from build123d import *

# Parameters (mm, degrees)
SKETCH1_W           = 48.5
SKETCH1_H           = 28
SKETCH1_W_2         = 40.5
SKETCH1_H_2         = 20
BOSS_EXTRUDE1_DEPTH = 40
SKETCH2_W           = 48.5
SKETCH2_H           = 28
BOSS_EXTRUDE2_DEPTH = 7
SKETCH3_W           = 15
SKETCH3_H           = 15
CUT_EXTRUDE1_DEPTH  = 10
SKETCH4_W           = 48.5
SKETCH4_H           = 58.5
BOSS_EXTRUDE3_DEPTH = 6
SKETCH4_3_W         = 48.5
SKETCH4_3_H         = 10
BOSS_EXTRUDE4_DEPTH = 35
SKETCH5_W           = 10
SKETCH5_H           = 10
BOSS_EXTRUDE5_DEPTH = 30.5


with BuildPart() as part:
    # Sketch1 → Boss-Extrude1 (new body)
    with BuildSketch(Plane(origin=(0, 0, -17.55), x_dir=(-1, 0, 0), z_dir=(0, 0, -1))):
        with Locations((-10.25, 0)):
            Rectangle(SKETCH1_W, SKETCH1_H)
        with Locations((-10.25, 0)):
            Rectangle(SKETCH1_W_2, SKETCH1_H_2, mode=Mode.SUBTRACT)
    extrude(amount=BOSS_EXTRUDE1_DEPTH)

    # Sketch2 → Boss-Extrude2 (add)
    with BuildSketch(Plane(origin=(0, 0, -57.55), x_dir=(-1, 0, 0), z_dir=(0, 0, -1))):
        with Locations((-10.25, 0)):
            Rectangle(SKETCH2_W, SKETCH2_H)
    extrude(amount=-BOSS_EXTRUDE2_DEPTH)

    # Sketch3 → Cut-Extrude1 (cut)
    with BuildSketch(Plane(origin=(34.5, 0, 0), x_dir=(0, 0, -1), z_dir=(1, 0, 0))):
        with Locations((48.05, 0)):
            Rectangle(SKETCH3_W, SKETCH3_H)
    extrude(amount=-CUT_EXTRUDE1_DEPTH, mode=Mode.SUBTRACT)

    # Sketch4 → Boss-Extrude3 (add)
    with BuildSketch(Plane(origin=(0, 0, -57.55), x_dir=(-1, 0, 0), z_dir=(0, 0, -1))):
        with Locations((-10.25, 15.25)):
            Rectangle(SKETCH4_W, SKETCH4_H)
    extrude(amount=BOSS_EXTRUDE3_DEPTH)

    # Sketch4<3> → Boss-Extrude4 (add)
    with BuildSketch(Plane(origin=(0, 0, -57.55), x_dir=(-1, 0, 0), z_dir=(0, 0, -1))):
        with Locations((-10.25, 39.5)):
            Rectangle(SKETCH4_3_W, SKETCH4_3_H)
    extrude(amount=BOSS_EXTRUDE4_DEPTH)

    # Sketch5 → Boss-Extrude5 (add)
    with BuildSketch(Plane.XZ.offset(-14)):
        with Locations((-9, -22.55)):
            Rectangle(SKETCH5_W, SKETCH5_H)
        with Locations((29.5, -22.55)):
            Rectangle(SKETCH5_W, SKETCH5_H)
    extrude(amount=-BOSS_EXTRUDE5_DEPTH)


solid = part.part
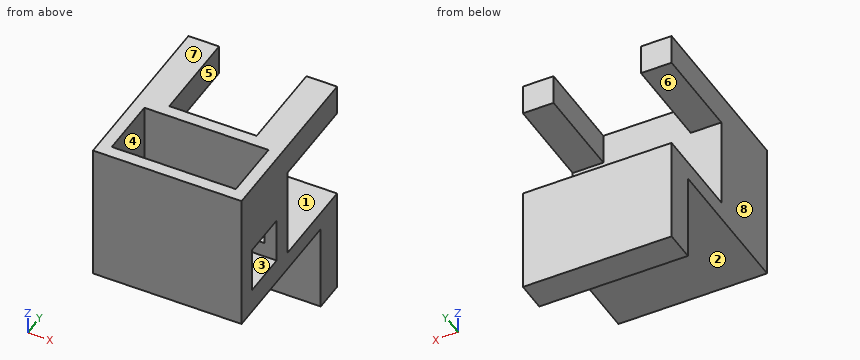
Work out the finished part from the listing and answer in its coordinate system (mm). Face numbers are marked on the shaded views. A direction names the side the tool comes from. Coordinates: 2 decimals unless noted, no trailing zeros. Loops run counter-clockwise (first coordinate to the right, second up) from the corner with the lowest first, then second, coordinate; pieces in that order, holes last. Notation, with made-up numbers: (36.25, 88.5) -> (47.25, 88.5) arc R19 ccw to (47.25, 93.5) -> close; hole circle Ø6 at (0, 74.5). An arc over 180 degrees is marked (long way). Write each question's results on one line, items separated by ' | '. Start each with the question number.
1) Find section A-A on y = 2. Determine the outline of the cut face in (x, z).
2) Find section D-D on x = 1. Determine the outline of the cut face in (y, z), then the cut area to 3 significant figures.
3) Find section C-C on y = 19.5. Determine the outline of the cut face in (x, z).
4) For the marked faces 1, 2, 3, 4 and 5, determine the directions among +Z, -Z, +X, -X, +Y, -Y from which every point of the face is accessible in a straight line to the end or side of a thin tool.
5) Consider line 1 along Y through (x, z) = (11.5, -43.5); line 2 along Z through (x, y) = (31.5, 37.5); line 3 along Y through (x, z) = (30, -26). Determine where each line is inside the solid, lowest interval first.
6) Find section B-B on z = -34.5. Determine the outline of the cut face in (x, y).
7) Flat-ended cylindrical pins translate along their axes: P1, Ø1.5, axis at y = 2, z = -52, coming from the +X side; P2, Ø8, axis at x = -8.5, y = 24.5, coming from the -Z side; P3, Ø1, axis at x = 24.5, y = -7.5, coming from the +Z side. Find the tip coordinate at first contact, or state that the pin passes through.
8) The mould has two halves that part along Z. Classify the marked faces 6, 7 and 8: pulls with the +Z half, pulls with the -Z half, needs draft (parallel to the pull), parting line crosses it, or undercut.
Response values:
1) outline: (-14, -63.55) -> (34.5, -63.55) -> (34.5, -55.55) -> (24.5, -55.55) -> (24.5, -50.55) -> (-10, -50.55) -> (-10, -17.55) -> (-14, -17.55) -> close; (30.5, -40.55) -> (34.5, -40.55) -> (34.5, -17.55) -> (30.5, -17.55) -> close
2) outline: (-14, -63.55) -> (34.5, -63.55) -> (34.5, -92.55) -> (44.5, -92.55) -> (44.5, -57.55) -> (14, -57.55) -> (14, -17.55) -> (10, -17.55) -> (10, -50.55) -> (-10, -50.55) -> (-10, -17.55) -> (-14, -17.55) -> close | area: 1,100 mm^2
3) outline: (-14, -63.55) -> (34.5, -63.55) -> (34.5, -57.55) -> (-14, -57.55) -> close; (-14, -27.55) -> (-4, -27.55) -> (-4, -17.55) -> (-14, -17.55) -> close; (24.5, -27.55) -> (34.5, -27.55) -> (34.5, -17.55) -> (24.5, -17.55) -> close
4) face 1: +X, -X, +Y | face 2: -Z, +X, -X, -Y | face 3: +X | face 4: +Z | face 5: +Z, +Y
5) line 1: y = -14 to -10, 10 to 14 | line 2: z = -92.55 to -57.55, -27.55 to -17.55 | line 3: y = -14 to -10, 10 to 44.5
6) outline: (-14, -14) -> (34.5, -14) -> (34.5, 14) -> (-14, 14) -> close; hole (-10, -10) -> (30.5, -10) -> (30.5, 10) -> (-10, 10) -> close
7) P1: stops at x = 24.5 | P2: stops at z = -63.55 | P3: stops at z = -50.55
8) face 6: undercut | face 7: pulls with the +Z half | face 8: needs draft
